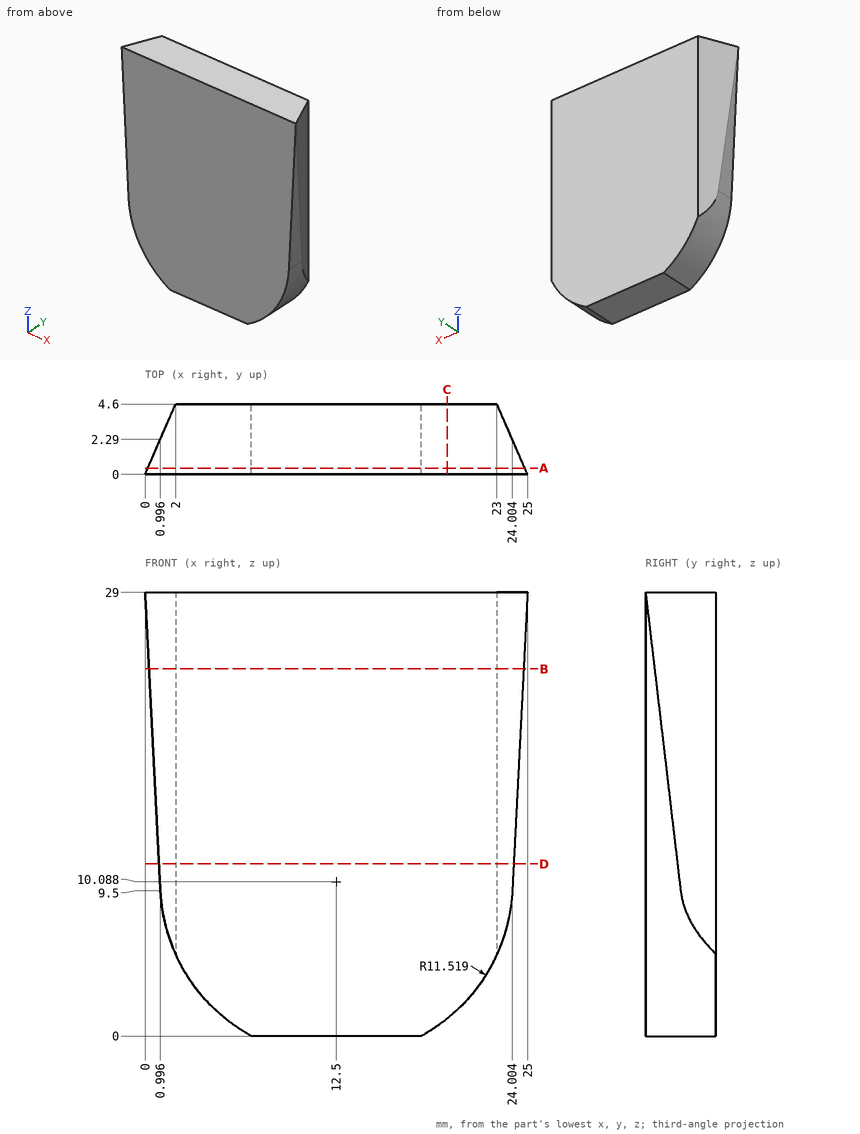
Check sheet for the drawn part. Datum: minimum x, y, z corner. Units: mm. Round coordinates to 2 decimals unless told otherwise and drop trailing zeros. Loops run counter-clockwise (first coordinate to the right, second up) from the corner with the lowest first, then second, coordinate; pieces in that order, holes last.
Item 1: Cross-section at B-B on z = 24. Record the boundary of the cut face in (x, y) (1 decimal), then the cut area to 3 significant figures.
Item 2: Cross-section at D-D on z = 11.25. Record the boundary of the cut face in (x, y) (1 decimal), then the cut area to 3 significant figures.
Item 3: Thickness scan on line 1 (X direction, y = 0.8, z = 4.5) (1 decimal); line 2 (X direction, y = 2.2, z = 14.25) (1 decimal); line 3 (Z direction, x = 2.5, y = 4). Record the ranges inside material, lowest first.
Item 4: Cross-section at A-A on y = 0.4. Record the boundary of the cut face in (x, z) (1 decimal).
Item 5: Cross-section at C-C on x = 19.75. Record the boundary of the cut face in (y, z), then the cut area to 3 significant figures.
Item 6: Gauge pin test, flat ends, axial feed: pin 1 (2 mm diameter, centred on y = 3, z = 15, fed in from +X); pin 2 (2 mm diameter, centred on x = 4, y = 1, fed in from -Z) (1 decimal). Record the tip position at first contact, or that the pin passes through.
Answer sheet:
1. outline: (0.3, 0) - (24.7, 0) - (24.7, 0.6) - (23, 4.6) - (2, 4.6) - (0.3, 0.6) - close
1. area: 106 mm2
2. outline: (0.9, 0) - (24.1, 0) - (24.1, 2.1) - (23, 4.6) - (2, 4.6) - (0.9, 2.1) - close
2. area: 104 mm2
3. line 1: x = 2.4 to 22.6
3. line 2: x = 1 to 24
3. line 3: z = 4.37 to 29
4. outline: (0.2, 25.6) - (1, 9.5) arc R11.5 ccw to (6.9, 0) - (18.1, 0) arc R11.5 ccw to (24, 9.5) - (24.8, 25.6) - (24.8, 29) - (0.2, 29) - close
5. outline: (0, 1.14) - (4.6, 1.14) - (4.6, 29) - (0, 29) - close
5. area: 128 mm2
6. pin 1: stops at x = 24.13
6. pin 2: stops at z = 1.3
